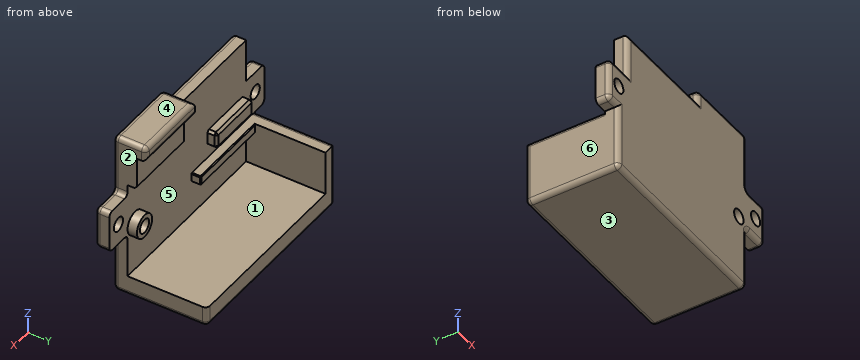
from build123d import *

# Parameters (mm, degrees)
ESQUISSE1_W         = 6
ESQUISSE1_H         = 9
ESQUISSE1_R         = 1.5
ESQUISSE1_W_2       = 39
ESQUISSE1_H_2       = 28
ESQUISSE1_R_2       = 1.55
BOSS_EXTRU_2_DEPTH  = 3
ESQUISSE2_W         = 12
ESQUISSE2_H         = 3.5
BOSS_EXTRU_3_DEPTH  = 2
CHANFREIN1_SIZE     = 0.5
ESQUISSE7_R         = 2.5
ESQUISSE7_R_2       = 1.5
BOSS_EXTRU_6_DEPTH  = 2
ESQUISSE5_W         = 18
ESQUISSE5_H         = 2
BOSS_EXTRU_7_DEPTH  = 5
CHANFREIN2_SIZE     = 0.2
ESQUISSE8_W         = 16
ESQUISSE8_H         = 7
BOSS_EXTRU_8_DEPTH  = 2
CHANFREIN3_SIZE     = 0.5
BOSS_EXTRU_9_DEPTH  = 20
ESQUISSE11_W        = 16
ESQUISSE11_H        = 3
BOSS_EXTRU_10_DEPTH = 7
CONG_1_R            = 1


with BuildPart() as part:
    # Esquisse1 → Boss.-Extru.2 (new body)
    # profile 1 of 3: a face of its own
    with BuildSketch(Plane(origin=(0, 0, 0), x_dir=(1, 0, 0), z_dir=(0, 1, 0))):
        with Locations((-22.5, 0)):
            Rectangle(ESQUISSE1_W, ESQUISSE1_H)
        with Locations(Location((-22.5, 0, 0), (0, 0, 270))):
            Circle(ESQUISSE1_R, mode=Mode.SUBTRACT)
    # profile 2 of 3: a face of its own
    with BuildSketch(Plane(origin=(0, 0, 0), x_dir=(1, 0, 0), z_dir=(0, 1, 0))):
        Rectangle(ESQUISSE1_W_2, ESQUISSE1_H_2)
        with Locations(Location((17, 3.25, 0), (0, 0, 270))):
            Circle(ESQUISSE1_R_2, mode=Mode.SUBTRACT)
    # profile 3 of 3: a face of its own
    with BuildSketch(Plane(origin=(0, 0, 0), x_dir=(1, 0, 0), z_dir=(0, 1, 0))):
        with Locations((22.5, 0)):
            Rectangle(ESQUISSE1_W, ESQUISSE1_H)
        with Locations(Location((22.5, 0, 0), (0, 0, 270))):
            Circle(ESQUISSE1_R, mode=Mode.SUBTRACT)
    extrude(amount=BOSS_EXTRU_2_DEPTH)

    # Esquisse2 → Boss.-Extru.3 (add)
    with BuildSketch(Plane(origin=(0, 3, 0), x_dir=(1, 0, 0), z_dir=(0, 1, 0))):
        with Locations((-12.765224295, 0)):
            Rectangle(ESQUISSE2_W, ESQUISSE2_H)
    extrude(amount=BOSS_EXTRU_3_DEPTH)

    # Chanfrein1
    chanfrein1_edges = [part.edges().sort_by_distance(p)[0] for p in [
        (-18.765224295, 4, -1.75),
        (-18.765224295, 4, 1.75),
        (-6.765224295, 4, 1.75),
        (-6.765224295, 4, -1.75),
        (-18.765224295, 5, 0),
        (-12.765224295, 5, 1.75),
        (-6.765224295, 5, 0),
        (-12.765224295, 5, -1.75),
    ]]
    chamfer(chanfrein1_edges, length=CHANFREIN1_SIZE)

    # Esquisse7 → Boss.-Extru.6 (add)
    with BuildSketch(Plane(origin=(0, 3, 0), x_dir=(1, 0, 0), z_dir=(0, 1, 0))):
        with Locations(Location((17, 3.25, 0), (0, 0, 270))):
            Circle(ESQUISSE7_R)
        with Locations(Location((17, 3.25, 0), (0, 0, 270))):
            Circle(ESQUISSE7_R_2, mode=Mode.SUBTRACT)
    extrude(amount=BOSS_EXTRU_6_DEPTH)

    # Esquisse5 → Boss.-Extru.7 (add)
    with BuildSketch(Plane.XZ):
        with Locations((-10.5, -5.5)):
            Rectangle(ESQUISSE5_W, ESQUISSE5_H)
    extrude(amount=-BOSS_EXTRU_7_DEPTH)

    # Chanfrein2
    chanfrein2_edges = [part.edges().sort_by_distance(p)[0] for p in [
        (-1.5, 4, -4.5),
        (-1.5, 5, -5.5),
        (-1.5, 4, -6.5),
        (-10.5, 5, -6.5),
        (-19.5, 5, -5.5),
        (-10.5, 5, -4.5),
    ]]
    chamfer(chanfrein2_edges, length=CHANFREIN2_SIZE)

    # Esquisse8 → Boss.-Extru.8 (add)
    with BuildSketch(Plane(origin=(0, 3, 0), x_dir=(1, 0, 0), z_dir=(0, 1, 0))):
        with Locations((11.5, -10.5)):
            Rectangle(ESQUISSE8_W, ESQUISSE8_H)
    extrude(amount=BOSS_EXTRU_8_DEPTH)

    # Chanfrein3
    chanfrein3_edges = [part.edges().sort_by_distance(p)[0] for p in [
        (3.5, 4, 7),
        (11.5, 5, 7),
        (3.5, 5, 10.5),
    ]]
    chamfer(chanfrein3_edges, length=CHANFREIN3_SIZE)

    # Esquisse9 → Boss.-Extru.9 (add)
    with BuildSketch(Plane.XZ):
        Polygon((-19.5, -14), (19.5, -14), (19.5, -18.364828329), (-22.5, -18.364828329), (-22.5, -4.5), (-19.5, -4.5), align=None)
    extrude(amount=-BOSS_EXTRU_9_DEPTH)

    # Esquisse11 → Boss.-Extru.10 (add)
    with BuildSketch(Plane.XZ):
        with Locations((11.5, 15.5)):
            Rectangle(ESQUISSE11_W, ESQUISSE11_H)
    extrude(amount=-BOSS_EXTRU_10_DEPTH)

    # Congé1
    cong_1_edges = [part.edges().sort_by_distance(p)[0] for p in [
        (-24, 0, -4.5),
        (-22.5, 11.5, -4.5),
        (19.5, 20, -16.182414164),
        (-1.5, 20, -18.364828329),
        (19.5, 10, -18.364828329),
        (-22.5, 20, -11.432414164),
        (-22.5, 10, -18.364828329),
        (-22.5, 0, -11.432414164),
        (-1.5, 0, -18.364828329),
        (19.5, 0, -11.432414164),
        (22.5, 0, -4.5),
        (11.5, 7, 14),
        (25.5, 0, 0),
        (19.5, 7, 15.5),
        (19.5, 3.5, 17),
        (11.5, 7, 17),
        (3.5, 3.5, 17),
        (11.5, 0, 17),
        (3.5, 0, 15.5),
        (22.5, 0, 4.5),
        (19.5, 0, 10.75),
        (-8, 0, 14),
        (-19.5, 0, 9.25),
        (-22.5, 0, 4.5),
        (-25.5, 0, 0),
        (-25.5, 1.5, -4.5),
        (19.5, 1.5, -4.5),
        (25.5, 1.5, -4.5),
        (25.5, 1.5, 4.5),
        (19.5, 1.5, 4.5),
        (-25.5, 1.5, 4.5),
    ]]
    fillet(cong_1_edges, radius=CONG_1_R)


solid = part.part
Input: part model. Units: mm. Frame: model coordinates. Face numbers are marked on the shaded views. A direction names the side the tool comes from. Round coordinates to 2 decimals unless told otherwise and drop trailing zeros. Order: outer loops, then holes, each group sorted by start corner. A loop starts at its lowest first (then second) coordinate and runs counter-clockwise, first axis right, second up. Notation, with made-up numbers: (24.25, 22) - (50.25, 22) arc R23 cw to (50.25, 57) - close; hole circle Ø5 at (-16, 69). An arc over 180 degrees is marked (long way). Answer as a JSON object with one key per item and string values. Group by question number.
(1) Material intervals for probe 1 along X at (y, z) = (2.15, 0); probe 2 along Z at (x, y) = (1, 11.5); probe 3 along X at (y, z) = (3.4, -3.25), sorted ascending. Write a range as from..to.
(2) Pin query (flat end, axial travel): P1, Ø0.8, axis at x = 12.5, z = 15.5, coming from the +Y side; P2, Ø2, axis at y = 15, z = -5.5, coming from the -X side; P3, Ø2, axis at x = 22.5, y = 2.5, coming from the -Z side; P4, Ø2.5, axis at x = 17, z = -3.25, coming from the -Y side. Return the tip coordinate at first contact, or that it passes through.
(3) Reachability of the marked faces 1, 2 and 3 from +Z, -Z, +X, -X, +Y, -Y: full face, straight path, thin tool, end or side. Return the list, or none.
(4) Cut plane A-A (z = 0). Return loops of the section in (x, y).
(5) Draft query along Z for the marked faces 4, 5 and 6. Return one class per face: released by +Z, released by -Z, zero draft, split by the parting line, or undercut.
(6) Cut plane B-B (y = 17). Return loops of the section in (x, z).
(7) Cut plane C-C (x = -17). Return loops of the section in (y, z).
Here are the results:
{
 "1": {"probe 1": "x = -25.5..-24, -21..21, 24..25.5", "probe 2": "z = -18.36..-14", "probe 3": "x = 14.5..15.5, 18.5..19.5"},
 "2": {"P1": "stops at y = 7", "P2": "stops at x = -22.5", "P3": "stops at z = -4.5", "P4": "passes through"},
 "3": {"face 1": "+X, +Y", "face 2": "+Z, +X, +Y, -Y", "face 3": "-Z, +X, -X, +Y, -Y"},
 "4": {"outline": "(-25.5, 1) arc R1 ccw to (-24.5, 0) - (-24, 0) - (-24, 3) - (-25.5, 3) - close; (-21, 0) - (21, 0) - (21, 3) - (-6.77, 3) - (-6.77, 4.5) - (-7.27, 5) - (-18.27, 5) - (-18.77, 4.5) - (-18.77, 3) - (-21, 3) - close; (24, 0) - (24.5, 0) arc R1 ccw to (25.5, 1) - (25.5, 3) - (24, 3) - close"},
 "5": {"face 4": "released by +Z", "face 5": "undercut", "face 6": "zero draft"},
 "6": {"outline": "(-22.5, -17.36) arc R1 ccw to (-21.5, -18.36) - (18.5, -18.36) arc R1 ccw to (19.5, -17.36) - (19.5, -14) - (-19.5, -14) - (-19.5, -4.5) - (-21.5, -4.5) arc R1 ccw to (-22.5, -5.5) - close"},
 "7": {"outline": "(0, -17.36) arc R1 ccw to (1, -18.36) - (19, -18.36) arc R1 ccw to (20, -17.36) - (20, -14) - (3, -14) - (3, -6.5) - (4.8, -6.5) - (5, -6.3) - (5, -4.7) - (4.8, -4.5) - (3, -4.5) - (3, -1.75) - (4.5, -1.75) - (5, -1.25) - (5, 1.25) - (4.5, 1.75) - (3, 1.75) - (3, 14) - (1, 14) arc R1 ccw to (0, 13) - close"}
}
